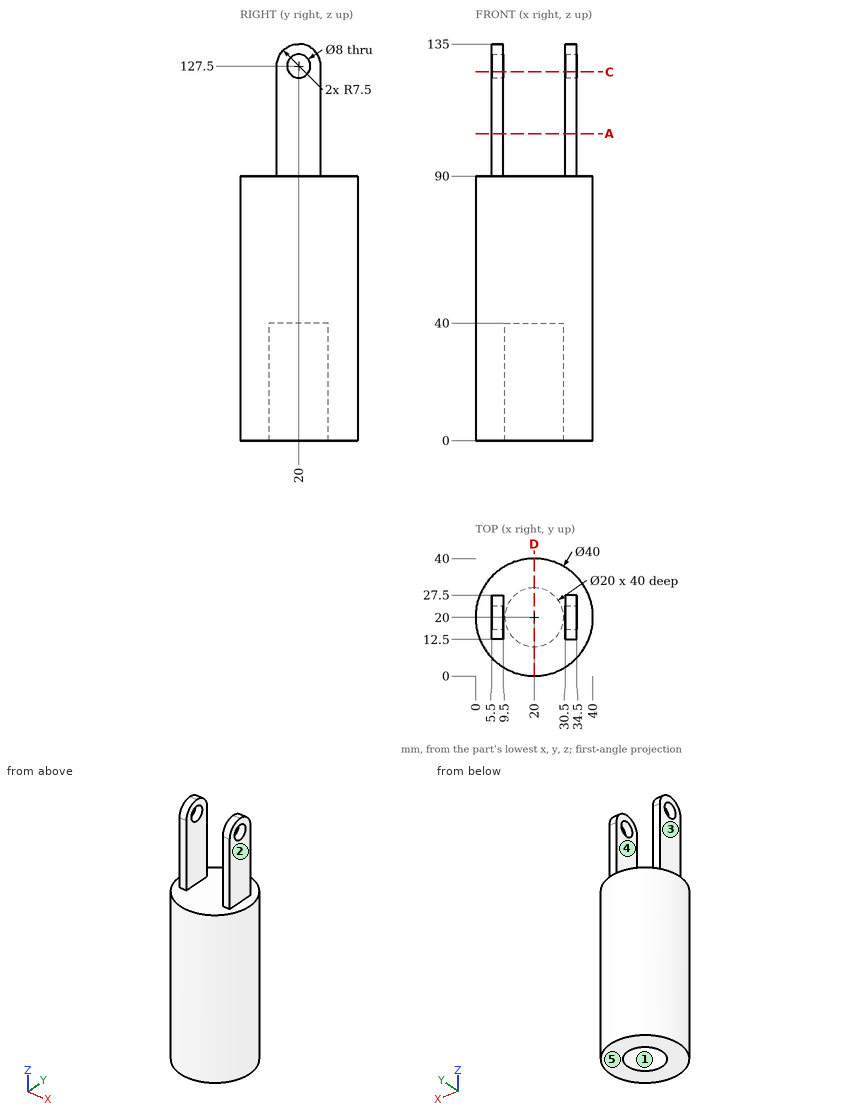
Can you work these out from the drawing? Everything is in mm from the part's minimum corner. A direction names the side the tool comes from. Give positions to 0.01 mm unless a question says otherwise; leave off trailing zeros. Loops run counter-clockwise (first coordinate to the right, second up) from the corner with the lowest first, then second, coordinate; pieces in that order, holes last. Notation, with made-up numbers: M 57,46 L 64,46 A25 cw 64,80 Z; hole C 65,21.25 d6. An arc over 180 degrees is marked long. Put each result on its own line as item: value. Start each with the question number.
(1) If we mould it in two halves opening along X, with no side actions, what happens to the marked faces 1, 2 and 3? For each: +X half, -X half, draft (parallel to the pull), parting line (faces both ways), or undercut.
(2) I need wall thicknesses on line 1 along X through (y, z) = (20.5, 18); line 2 along Z through (x, y) = (31, 20); line 3 along Z through (x, y) = (10.5, 33). Which ranges of each line are inside material? Lowest first, please. Write a range as [from, to].
(3) I want a section at D-D on x = 20. Please give me the cut outline in (y, z), then the cut area to 3 significant figures.
(4) For the marked faces 4 and 5, which set-ups out of +Z, -Z, +X, -X, +Y, -Y let a thin tool reach every point of the face, with its end or its side?
(5) I want a section at C-C on z = 125.5. Please give me the cut outline in (x, y).
(6) I want a section at A-A on z = 104.5. Please give me the cut outline in (x, y).
(7) Will these pins go through, and if not, where does the flat tip stop? pin 1 Ø2 at (x, z) = (7.5, 115) entering from -Y; pin 2 Ø16 at (x, y) = (20, 20) entering from +Z; pin 3 Ø7.5 at (y, z) = (18.5, 102) entering from +X.
Answer block:
1. face 1: undercut
1. face 2: +X half
1. face 3: -X half
2. line 1: [0.01, 10.01], [29.99, 39.99]
2. line 2: [0, 123.5], [131.5, 135]
2. line 3: [0, 90]
3. outline: M 0,0 L 10,0 L 10,40 L 30,40 L 30,0 L 40,0 L 40,90 L 0,90 Z
3. area: 2,800 mm^2
4. face 4: +Z, +Y, -Y
4. face 5: -Z, +X, -X, +Y, -Y
5. outline: M 5.5,12.5 L 9.5,12.5 L 9.5,16.54 L 5.5,16.54 Z; M 5.5,23.46 L 9.5,23.46 L 9.5,27.5 L 5.5,27.5 Z; M 30.5,12.5 L 34.5,12.5 L 34.5,16.54 L 30.5,16.54 Z; M 30.5,23.46 L 34.5,23.46 L 34.5,27.5 L 30.5,27.5 Z
6. outline: M 5.5,12.5 L 9.5,12.5 L 9.5,27.5 L 5.5,27.5 Z; M 30.5,12.5 L 34.5,12.5 L 34.5,27.5 L 30.5,27.5 Z
7. pin 1: y = 12.5
7. pin 2: z = 90
7. pin 3: x = 34.5
